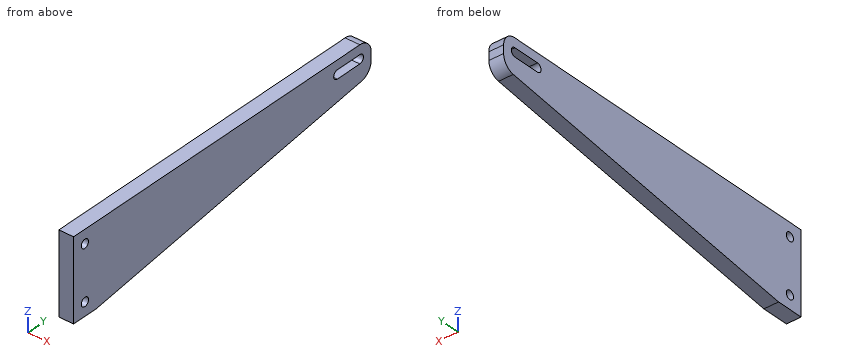
```python
from build123d import *

# Parameters (mm, degrees)
SKETCH1_R           = 1.6
BOSS_EXTRUDE1_DEPTH = 5.4864


with BuildPart() as part:
    # Sketch1 → Boss-Extrude1 (new body)
    with BuildSketch(Plane(origin=(0, 0, 0), x_dir=(0, 0, -1), z_dir=(1, 0, 0))):
        with BuildLine():
            Line((0, 0), (30, 0))
            Line((30, 0), (30, 10))
            Line((30, 10), (12.948355245, 127.716784747))
            ThreePointArc((12.948355245, 127.716784747), (11.272313881, 130.780471117), (8, 132))
            Line((8, 132), (5, 132))
            ThreePointArc((5, 132), (1.464466094, 130.535533906), (0, 127))
            Line((0, 127), (0, 0))
        make_face()
        with Locations((5, 5)):
            Circle(SKETCH1_R, mode=Mode.SUBTRACT)
        with Locations((25, 5)):
            Circle(SKETCH1_R, mode=Mode.SUBTRACT)
        with BuildLine():
            Line((3.4, 117), (3.4, 127))
            ThreePointArc((3.4, 127), (5, 128.6), (6.6, 127))
            Line((6.6, 127), (6.6, 117))
            ThreePointArc((6.6, 117), (5, 115.4), (3.4, 117))
        make_face(mode=Mode.SUBTRACT)
    extrude(amount=BOSS_EXTRUDE1_DEPTH)


solid = part.part
```
Model file for the job. Use its own axes, mm. Give positions to 0.01 mm unless a question says otherwise; leave off trailing zeros. Order: outer loops, then holes, each group sorted by start corner. A loop starts at its lowest first (then second) coordinate and runs counter-clockwise, first axis right, second up.
1) Saw through at A-A, the plane x = 2.75. Write the cut outline in (y, z), then the cut area to 3 significant figures.
2) Saw through at C-C, the plane y = 58.5. Write the cut outline in (x, z), then the cut area to 3 significant figures.
3) Wall check: probe 1 along Y at (x, z) = (4.2, -5); probe 2 along Y at (x, z) = (1.1, -4); probe 3 along Z at (x, y) = (0.9, 124.5). Give the ranges that are in metal, low to high.
4) Saw through at B-B, the plane z = -25. Write the cut outline in (x, y), then the cut area to 3 significant figures.
5) Pin check, flat tips, straight feed: pin 1 (1.6 mm diameter, centred on x = 3, y = 124.5, fed in from -Z); pin 2 (3 mm diameter, centred on y = 5, z = -25, fed in from +X). Stop position of each tip, or through.
6) Saw through at D-D, the plane y = 28. Write the cut outline in (x, z), then the cut area to 3 significant figures.
Computed:
1. outline: (0, -30) - (10, -30) - (127.72, -12.95) arc R5 ccw to (132, -8) - (132, -5) arc R5 ccw to (127, 0) - (0, 0) - close; hole circle Ø3.2 at (5, -25); hole circle Ø3.2 at (5, -5); hole (117, -6.6) - (127, -6.6) arc R1.6 ccw to (127, -3.4) - (117, -3.4) arc R1.6 ccw to start
1. area: 2,820 mm2
2. outline: (0, -22.97) - (5.49, -22.97) - (5.49, 0) - (0, 0) - close
2. area: 126 mm2
3. probe 1: y = 0 to 3.4, 6.6 to 115.4, 128.6 to 132
3. probe 2: y = 0 to 3.75, 6.25 to 115.75, 128.25 to 131.9
3. probe 3: z = -13.41 to -6.6, -3.4 to 0
4. outline: (0, 0) - (5.49, 0) - (5.49, 3.4) - (0, 3.4) - close; (0, 6.6) - (5.49, 6.6) - (5.49, 44.52) - (0, 44.52) - close
4. area: 227 mm2
5. pin 1: stops at z = -13.53
5. pin 2: passes through
6. outline: (0, -27.39) - (5.49, -27.39) - (5.49, 0) - (0, 0) - close
6. area: 150 mm2
